from build123d import *

# Parameters (mm, degrees)
F0_R     = 17
F1_DEPTH = 7
F3_D     = 6.8
F4_D     = 2.5


with BuildPart() as f1:
    # F0 (on Top) → F1 (new body)
    with BuildSketch(Plane.XY):
        Circle(F0_R)
    extrude(amount=F1_DEPTH)

    # F3 (through all)
    with Locations(Plane.XY.offset(7)):
        with Locations((0, 0)):
            Hole(F3_D / 2)

    # F4 (through all)
    with Locations(Plane.XY.offset(7)):
        with Locations((0, 12.5), (10.8253175473, -6.25), (-10.8253175473, -6.25)):
            Hole(F4_D / 2)


solid = f1.part
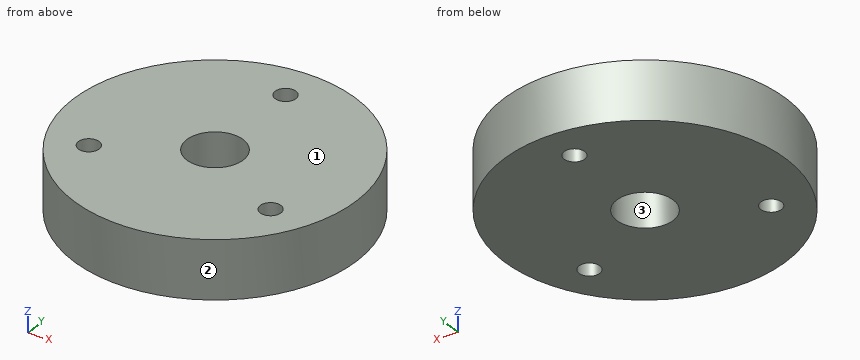
For this review, take the finished solid that the model builds, in its own axes (mm). Face numbers are marked on the shaded views. Round coordinates to 2 decimals unless told otherwise and drop trailing zeros. Order: outer loops, then holes, each group sorted by start corner. A loop starts at its lowest first (then second) coordinate and runs counter-clockwise, first axis right, second up. Notation, with made-up numbers: (19.25, 69) -> (62.25, 69) arc R32 cw to (62.25, 103) -> close; hole circle Ø1 at (73, -30). An arc over 180 degrees is marked (long way). Put each result on its own line as item: value.
Q1. Add section B-B on x = 0. Write out the cut boundary in (y, z).
Check result:
outline: (-17, 0) -> (-3.4, 0) -> (-3.4, 7) -> (-17, 7) -> close; (3.4, 0) -> (11.25, 0) -> (11.25, 7) -> (3.4, 7) -> close; (13.75, 0) -> (17, 0) -> (17, 7) -> (13.75, 7) -> close
Q2. Add section D-D on y = -6.25. Write out the cut boundary in (x, z), plus the area to 3 significant figures.
Check result:
outline: (-15.81, 0) -> (-12.08, 0) -> (-12.08, 7) -> (-15.81, 7) -> close; (-9.58, 0) -> (9.58, 0) -> (9.58, 7) -> (-9.58, 7) -> close; (12.08, 0) -> (15.81, 0) -> (15.81, 7) -> (12.08, 7) -> close
area: 186 mm2
Q3. Add section C-C on y = -1. Write out the cut boundary in (x, z), plus the area to 3 significant figures.
Check result:
outline: (-16.97, 0) -> (-3.25, 0) -> (-3.25, 7) -> (-16.97, 7) -> close; (3.25, 0) -> (16.97, 0) -> (16.97, 7) -> (3.25, 7) -> close
area: 192 mm2
Q4. Mouldability with a two-part tool opening along Y and no side actions: class the marked faces 1, 2 and 3 as pulls with the +Y half, pulls with the -Y half, needs draft (parallel to the pull), parting line crosses it, or undercut.
Check result:
face 1: needs draft
face 2: parting line crosses it
face 3: undercut
Q5. Add section A-A on z = 1.75. Write out the cut boundary in (x, y), plus the area to 3 significant figures.
Check result:
outline: circle Ø34 at (0, 0); hole circle Ø2.5 at (-10.83, -6.25); hole circle Ø6.8 at (0, 0); hole circle Ø2.5 at (0, 12.5); hole circle Ø2.5 at (10.83, -6.25)
area: 857 mm2
Q6. For probe 1 along Y at (x, z) = (0, 4); probe 2 along X at (y, z) = (14.5, 5); probe 3 along Y at (x, z) = (-3, 5.25), list the stretches that pass through material, from the lowest coordinate up. Write a range as [from, to].
Check result:
probe 1: [-17, -3.4], [3.4, 11.25], [13.75, 17]
probe 2: [-8.87, 8.87]
probe 3: [-16.73, -1.6], [1.6, 16.73]
Q7. Insertion check: pin 1 Ø3 at (x, y) = (-10.83, -6.25) entering from +Z; pin 2 Ø1 at (x, z) = (-11.5, 1.5) entering from +Y; pin 3 Ø6 at (x, y) = (0, 0) entering from -Z; pin 4 Ø3 at (x, z) = (-11, 5.5) entering from -Y. Each pin has a flat end and moves straight along its axis. Give the tip position at first contact, or say it passes through.
Check result:
pin 1: z = 7
pin 2: y = 12.96
pin 3: through
pin 4: y = -14.1
